Build history of the part. All positions in model axes, mm. A direction names the side the tool comes from. Give positions to 0.01 mm unless a question says otherwise; leave off trailing zeros. Loops run counter-clockwise (first coordinate to the right, second up) from the corner with the lowest first, then second, coordinate; pieces in that order, holes last. Notation, with made-up numbers: (-26, 0.25) -> (13, 0.25) arc R13 ccw to (13, 16.25) -> close; hole circle Ø3 at (15.5, -19.5). An arc over 180 degrees is marked (long way). Answer as a JSON object with one key per item and string values. Group by question number.
from build123d import *

# Parameters (mm, degrees)
BOSS_EXTRUDE1_DEPTH = 4.3
SKETCH3_W           = 8
SKETCH3_H           = 2
CUT_EXTRUDE1_DEPTH  = 4.3
SKETCH4_W           = 11
SKETCH4_H           = 12
CUT_EXTRUDE2_DEPTH  = 3.3


with BuildPart() as part:
    # Sketch2 → Boss-Extrude1 (new body)
    with BuildSketch(Plane.XY):
        Polygon((4, -15.4), (-15.7, -15.4), (-15.7, -8.4), (-22.9, -8.4), (-22.9, 15.4), (22.9, 15.4), (22.9, -8.4), (15.7, -8.4), (15.7, -15.4), align=None)
    extrude(amount=-BOSS_EXTRUDE1_DEPTH)

    # Sketch3 → Cut-Extrude1 (cut)
    with BuildSketch(Plane.XY):
        with Locations((0, -14.5)):
            Rectangle(SKETCH3_W, SKETCH3_H)
    extrude(amount=-CUT_EXTRUDE1_DEPTH, mode=Mode.SUBTRACT)

    # Sketch4 → Cut-Extrude2 (cut)
    with BuildSketch(Plane(origin=(0, 0, -4.3), x_dir=(-1, 0, 0), z_dir=(0, 0, -1))):
        with Locations((0, -7.5)):
            Rectangle(SKETCH4_W, SKETCH4_H)
    extrude(amount=-CUT_EXTRUDE2_DEPTH, mode=Mode.SUBTRACT)


solid = part.part
(1) Saw through at D-D on x = -17. List the corners of the cut face in (y, z).
(2) Saw through at B-B on x = -5. List the corners of the cut face in (y, z).
(3) 3-axis set-ups, long thin cutter, end or side, ignore diameter. For faces 4 (the flat face through (0, -7, -1)), 5 (the flat face through (-15.7, -12, -2)), 6 (the flat face through (19, -8.4, -2)), 7 (the flat face through (-4, -14, -2)): which of +Z, -Z, +X, -X, +Y, -Y reach the whole face in a straight line?
(4) Saw through at A-A on z = -2.5. List the corners of the cut face in (x, y), plus the area to 3 significant figures.
(5) Pull direction Y, two halves, no side cores. Call faces 1 (the flat face through (-5, -13.5, -3)), 2 (the flat face through (15.7, -12, -2)), 3 (the flat face through (-19, -8.4, -2)): pulls with the +Y half, pulls with the -Y half, needs draft (parallel to the pull), parting line crosses it, or undercut.
(6) Probe line 1 along X through (y, z) = (-9.5, -2.45); line 2 along Y through (x, z) = (17, -3.05); line 3 along Z through (x, y) = (3.5, -12). List the from-to ranges inside material, lowest first. Write a range as [from, to].
(7) Pin check, flat tips, straight feed: pin 1 (3.5 mm diameter, centred on x = -2.5, y = -4.5, fed in from -Z); pin 2 (2 mm diameter, centred on x = 19.5, z = -2, fed in from -Y); pin 3 (2 mm diameter, centred on y = -11.5, z = -3, fed in from -X). Stop position of each tip, or through.
(8) Saw through at C-C on y = -9. List the corners of the cut face in (x, z).
Calculated:
{
 "1": {"outline": "(-8.4, -4.3) -> (15.4, -4.3) -> (15.4, 0) -> (-8.4, 0) -> close"},
 "2": {"outline": "(-15.4, -4.3) -> (-13.5, -4.3) -> (-13.5, -1) -> (-1.5, -1) -> (-1.5, -4.3) -> (15.4, -4.3) -> (15.4, 0) -> (-15.4, 0) -> close"},
 "3": {"face 4": "-Z", "face 5": "+Z, -Z, -X, -Y", "face 6": "+Z, -Z, +X, -Y", "face 7": "+Z, -Z, -Y"},
 "4": {"outline": "(-22.9, -8.4) -> (-15.7, -8.4) -> (-15.7, -15.4) -> (-4, -15.4) -> (-4, -13.5) -> (-5.5, -13.5) -> (-5.5, -1.5) -> (5.5, -1.5) -> (5.5, -13.5) -> (4, -13.5) -> (4, -15.4) -> (15.7, -15.4) -> (15.7, -8.4) -> (22.9, -8.4) -> (22.9, 15.4) -> (-22.9, 15.4) -> close", "area": "1,160 mm^2"},
 "5": {"face 1": "undercut", "face 2": "needs draft", "face 3": "pulls with the -Y half"},
 "6": {"line 1": "x = [-15.7, -5.5], [5.5, 15.7]", "line 2": "y = [-8.4, 15.4]", "line 3": "z = [-1, 0]"},
 "7": {"pin 1": "stops at z = -1", "pin 2": "stops at y = -8.4", "pin 3": "stops at x = -15.7"},
 "8": {"outline": "(-15.7, -4.3) -> (-5.5, -4.3) -> (-5.5, -1) -> (5.5, -1) -> (5.5, -4.3) -> (15.7, -4.3) -> (15.7, 0) -> (-15.7, 0) -> close"}
}
